Could you check a few things on this model? Use its own coordinates, in mm. A direction names the side the tool comes from. Round coordinates to 2 decimals unless told otherwise and drop trailing zeros. Write each loop counter-clockwise with the first axis right and the second up, starting at its lowest first coordinate (ties: lowest second). Pieces come first, ordered by that corner, then holes.
```python
from build123d import *

# Parameters (mm, degrees)
SKETCH1_R           = 3.25
SKETCH1_R_2         = 2
BOSS_EXTRUDE1_DEPTH = 5
FILLET2_R           = 10


with BuildPart() as part:
    # Sketch1 → Boss-Extrude1 (new body)
    with BuildSketch(Plane(origin=(0, 0, 0), x_dir=(1, 0, 0), z_dir=(0, 1, 0))):
        with BuildLine():
            ThreePointArc((171.761705084, -2.5), (172.431578065, 0), (171.761705084, 2.5))
            Line((171.761705084, 2.5), (88.045916051, 147.5))
            ThreePointArc((88.045916051, 147.5), (86.215789032, 149.330127019), (83.715789032, 150))
            Line((83.715789032, 150), (-83.715789032, 150))
            ThreePointArc((-83.715789032, 150), (-86.215789032, 149.330127019), (-88.045916051, 147.5))
            Line((-88.045916051, 147.5), (-171.761705084, 2.5))
            ThreePointArc((-171.761705084, 2.5), (-172.431578065, 0), (-171.761705084, -2.5))
            Line((-171.761705084, -2.5), (-88.045916051, -147.5))
            ThreePointArc((-88.045916051, -147.5), (-86.215789032, -149.330127019), (-83.715789032, -150))
            Line((-83.715789032, -150), (83.715789032, -150))
            ThreePointArc((83.715789032, -150), (86.215789032, -149.330127019), (88.045916051, -147.5))
            Line((88.045916051, -147.5), (171.761705084, -2.5))
        make_face()
        with Locations(Location((-80, -138.564064606, 0), (0, 0, 270))):
            Circle(SKETCH1_R, mode=Mode.SUBTRACT)
        with BuildLine():
            Line((20.920144878, -56.23475383), (59.178402592, -122.5))
            ThreePointArc((59.178402592, -122.5), (59.178402592, -127.5), (54.848275573, -130))
            Line((54.848275573, -130), (-54.848275573, -130))
            ThreePointArc((-54.848275573, -130), (-59.178402592, -127.5), (-59.178402592, -122.5))
            Line((-59.178402592, -122.5), (-20.920144878, -56.23475383))
            ThreePointArc((-20.920144878, -56.23475383), (0, -60), (20.920144878, -56.23475383))
        make_face(mode=Mode.SUBTRACT)
        with BuildLine():
            Line((-38.240652953, -46.23475383), (-76.498910668, -112.5))
            ThreePointArc((-76.498910668, -112.5), (-80.829037687, -115), (-85.159164705, -112.5))
            Line((-85.159164705, -112.5), (-140.007440278, -17.5))
            ThreePointArc((-140.007440278, -17.5), (-140.007440278, -12.5), (-135.67731326, -10))
            Line((-135.67731326, -10), (-59.160797831, -10))
            ThreePointArc((-59.160797831, -10), (-51.961524227, -30), (-38.240652953, -46.23475383))
        make_face(mode=Mode.SUBTRACT)
        with Locations(Location((-160, 0, 0), (0, 0, 270))):
            Circle(SKETCH1_R, mode=Mode.SUBTRACT)
        with Locations(Location((0, -52, 0), (0, 0, 270))):
            Circle(SKETCH1_R_2, mode=Mode.SUBTRACT)
        with Locations(Location((-52, 0, 0), (0, 0, 270))):
            Circle(SKETCH1_R_2, mode=Mode.SUBTRACT)
        with Locations(Location((80, -138.564064606, 0), (0, 0, 270))):
            Circle(SKETCH1_R, mode=Mode.SUBTRACT)
        with Locations(Location((52, 0, 0), (0, 0, 270))):
            Circle(SKETCH1_R_2, mode=Mode.SUBTRACT)
        with BuildLine():
            ThreePointArc((85.159164705, -112.5), (80.829037687, -115), (76.498910668, -112.5))
            Line((76.498910668, -112.5), (38.240652953, -46.23475383))
            ThreePointArc((38.240652953, -46.23475383), (51.961524227, -30), (59.160797831, -10))
            Line((59.160797831, -10), (135.67731326, -10))
            ThreePointArc((135.67731326, -10), (140.007440278, -12.5), (140.007440278, -17.5))
            Line((140.007440278, -17.5), (85.159164705, -112.5))
        make_face(mode=Mode.SUBTRACT)
        with BuildLine():
            Line((-59.160797831, 10), (-135.67731326, 10))
            ThreePointArc((-135.67731326, 10), (-140.007440278, 12.5), (-140.007440278, 17.5))
            Line((-140.007440278, 17.5), (-85.159164705, 112.5))
            ThreePointArc((-85.159164705, 112.5), (-80.829037687, 115), (-76.498910668, 112.5))
            Line((-76.498910668, 112.5), (-38.240652953, 46.23475383))
            ThreePointArc((-38.240652953, 46.23475383), (-51.961524227, 30), (-59.160797831, 10))
        make_face(mode=Mode.SUBTRACT)
        with Locations(Location((0, 52, 0), (0, 0, 270))):
            Circle(SKETCH1_R_2, mode=Mode.SUBTRACT)
        with BuildLine():
            Line((59.178402592, 122.5), (20.920144878, 56.23475383))
            ThreePointArc((20.920144878, 56.23475383), (0, 60), (-20.920144878, 56.23475383))
            Line((-20.920144878, 56.23475383), (-59.178402592, 122.5))
            ThreePointArc((-59.178402592, 122.5), (-59.178402592, 127.5), (-54.848275573, 130))
            Line((-54.848275573, 130), (54.848275573, 130))
            ThreePointArc((54.848275573, 130), (59.178402592, 127.5), (59.178402592, 122.5))
        make_face(mode=Mode.SUBTRACT)
        with Locations(Location((-80, 138.564064606, 0), (0, 0, 270))):
            Circle(SKETCH1_R, mode=Mode.SUBTRACT)
        with Locations(Location((160, 0, 0), (0, 0, 270))):
            Circle(SKETCH1_R, mode=Mode.SUBTRACT)
        with BuildLine():
            Line((135.67731326, 10), (59.160797831, 10))
            ThreePointArc((59.160797831, 10), (51.961524227, 30), (38.240652953, 46.23475383))
            Line((38.240652953, 46.23475383), (76.498910668, 112.5))
            ThreePointArc((76.498910668, 112.5), (80.829037687, 115), (85.159164705, 112.5))
            Line((85.159164705, 112.5), (140.007440278, 17.5))
            ThreePointArc((140.007440278, 17.5), (140.007440278, 12.5), (135.67731326, 10))
        make_face(mode=Mode.SUBTRACT)
        with Locations(Location((80, 138.564064606, 0), (0, 0, 270))):
            Circle(SKETCH1_R, mode=Mode.SUBTRACT)
    extrude(amount=BOSS_EXTRUDE1_DEPTH)

    # Fillet2
    fillet2_edges = [part.edges().sort_by_distance(p)[0] for p in [
        (-59.160797831, 2.5, -10),
        (-59.160797831, 2.5, 10),
        (-38.240652953, 2.5, 46.23475383),
        (-20.920144878, 2.5, 56.23475383),
        (20.920144878, 2.5, 56.23475383),
        (38.240652953, 2.5, 46.23475383),
        (59.160797831, 2.5, 10),
        (59.160797831, 2.5, -10),
        (38.240652953, 2.5, -46.23475383),
        (20.920144878, 2.5, -56.23475383),
        (-20.920144878, 2.5, -56.23475383),
        (-38.240652953, 2.5, -46.23475383),
    ]]
    fillet(fillet2_edges, radius=FILLET2_R)


solid = part.part
```
Q1. Imagine slicing it at B-B, the plane y = 2.8. Count the separate pieces of the cut face and the enclosed holes in it, then the cut area to 3 significant figures.
Q2. I'm going to push flat-ended pins straight in: pin 1 Ø2.5 at (x, y) = (97.5, 1.5) entering from -Z; pin 2 Ø2.5 at (x, y) = (107, 2.5) entering from +Z; pin 3 Ø1 at (x, y) = (91.5, 2.5) entering from -Z. Where does each tip first touch, or does it pass through?
Q3. We'd pull the mould along Z, two halves only. Please class faces 3 (the flat face through (-129.32, 2.46, -76.01)), 4 (the cylindrical face through (-52.06, 2.46, 29.83)), 5 (the flat face through (-59.59, 2.46, -83.21)), 6 (the flat face through (-2, 5, -2)): pulls with the +Z half, pulls with the -Z half, needs draft (parallel to the pull), parting line crosses it, or undercut.
Q4. On a 3-axis mill with a long thin cutter (end or side, diameter ignored), from which of +Z, -Z, +X, -X, +Y, -Y can I reach the whole of each face in a straight line? I mean faces 1 (the flat face through (-2, 0, -2)), 2 (the cylindrical face through (-61.03, 2.54, 12.04)). Say none if no direction works.
Q5. If I drill on L1, parallel to Z at x = -59, y = 1.65; L2, parallel to X at y = 4, z = -111.5; L3, parallel to Z at x = -90, y = 1.3, over which ranges is the centre line in solid material (lowest first)?
Q6. Imagine slicing it at A-A, the plane z = -72. Write out the boundary of the cut face in (x, y).
Results found:
1. separate pieces: 1
1. enclosed holes: 16
1. area: 41,300 mm2
2. pin 1: stops at z = -133.29
2. pin 2: stops at z = 116.84
2. pin 3: stops at z = -142.38
3. face 3: pulls with the -Z half
3. face 4: undercut
3. face 5: undercut
3. face 6: needs draft
4. face 1: +Z, -Z, +X, -X, -Y
4. face 2: +Y, -Y
5. L1: z = -150 to -127.79, -122.19 to -82.19, -14.11 to 14.11, 82.19 to 122.19, 127.79 to 150
5. L2: x = -108.83 to -85.74, -75.92 to -52.83, 52.83 to 75.92, 85.74 to 108.83
5. L3: z = -144.12 to -104.12, -10 to 10, 104.12 to 144.12
6. outline: (-131.64, 0) - (-108.54, 0) - (-108.54, 5) - (-131.64, 5) - close; (-53.12, 0) - (-30.02, 0) - (-30.02, 5) - (-53.12, 5) - close; (30.02, 0) - (53.12, 0) - (53.12, 5) - (30.02, 5) - close; (108.54, 0) - (131.64, 0) - (131.64, 5) - (108.54, 5) - close
